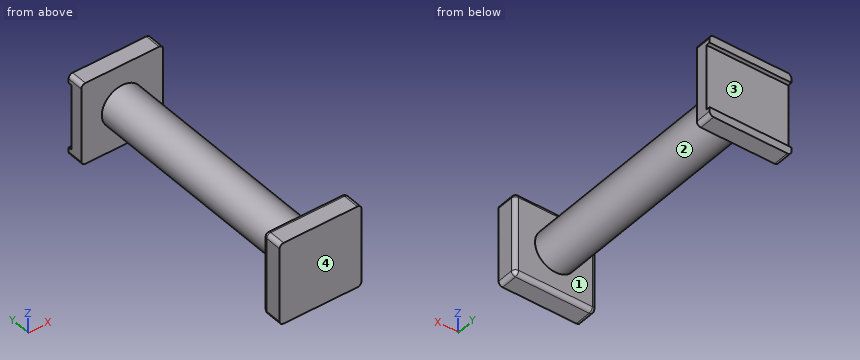
from build123d import *

# Parameters (mm, degrees)
SKETCH_1_W      = 20
SKETCH_1_H      = 20
EXTRUDE_1_DEPTH = 5
SKETCH_2_R      = 5
EXTRUDE_2_DEPTH = 57
SKETCH_4_W      = 20
SKETCH_4_H      = 20
EXTRUDE_3_DEPTH = 3
SKETCH_5_W      = 20
SKETCH_5_H      = 2
EXTRUDE_4_DEPTH = 1
SKETCH_6_W      = 20
SKETCH_6_H      = 2
EXTRUDE_5_DEPTH = 1
FILLET_1_R      = 1
FILLET_2_R      = 1
FILLET_3_R      = 1


with BuildPart() as part:
    # 草图1 → 凸台-拉伸1 (new body)
    with BuildSketch(Plane(origin=(0, 0, 0), x_dir=(1, 0, 0), z_dir=(0, 1, 0))):
        with Locations((-10, 10)):
            Rectangle(SKETCH_1_W, SKETCH_1_H)
    extrude(amount=EXTRUDE_1_DEPTH)

    # 草图2 → 凸台-拉伸2 (add)
    with BuildSketch(Plane(origin=(0, 5, 0), x_dir=(1, 0, 0), z_dir=(0, 1, 0))):
        with Locations(Location((-10, 10, 0), (0, 0, 90))):
            Circle(SKETCH_2_R)
    extrude(amount=EXTRUDE_2_DEPTH)

    # 草图4 → 凸台-拉伸3 (add)
    with BuildSketch(Plane(origin=(0, 62, 0), x_dir=(1, 0, 0), z_dir=(0, 1, 0))):
        with Locations((-10, 10)):
            Rectangle(SKETCH_4_W, SKETCH_4_H)
    extrude(amount=EXTRUDE_3_DEPTH)

    # 草图5 → 凸台-拉伸4 (add)
    with BuildSketch(Plane(origin=(0, 65, 0), x_dir=(1, 0, 0), z_dir=(0, 1, 0))):
        with Locations((-10, 19)):
            Rectangle(SKETCH_5_W, SKETCH_5_H)
    extrude(amount=EXTRUDE_4_DEPTH)

    # 草图6 → 凸台-拉伸5 (add)
    with BuildSketch(Plane(origin=(0, 65, 0), x_dir=(1, 0, 0), z_dir=(0, 1, 0))):
        with Locations((-10, 1)):
            Rectangle(SKETCH_6_W, SKETCH_6_H)
    extrude(amount=EXTRUDE_5_DEPTH)

    # 圆角1
    fillet_1_edges = [part.edges().sort_by_distance(p)[0] for p in [
        (0, 64, 0),
    ]]
    fillet(fillet_1_edges, radius=FILLET_1_R)

    # 圆角2
    fillet_2_edges = [part.edges().sort_by_distance(p)[0] for p in [
        (-20, 64, -20),
        (-20, 64, 0),
        (0, 64, -20),
    ]]
    fillet(fillet_2_edges, radius=FILLET_2_R)

    # 圆角3
    fillet_3_edges = [part.edges().sort_by_distance(p)[0] for p in [
        (-20, 5, -10),
        (-10, 5, 0),
        (0, 5, -10),
        (0, 2.5, 0),
        (-20, 2.5, 0),
        (-20, 2.5, -20),
        (0, 2.5, -20),
        (-10, 5, -20),
    ]]
    fillet(fillet_3_edges, radius=FILLET_3_R)


solid = part.part
Build history of the part. All positions in model axes, mm. Face numbers are marked on the shaded views. Give positions to 0.01 mm unless a question says otherwise; leave off trailing zeros. Order: outer loops, then holes, each group sorted by start corner. A loop starts at its lowest first (then second) coordinate and runs counter-clockwise, first axis right, second up. Notation, with made-up numbers: M -4.5,65.25 L 19.5,65.25 A25 cw 19.5,90.25 Z; hole C 54.5,-6 d8. An arc over 180 degrees is marked long. Put each result on its own line as item: value.
Item 1: Pull direction Y, two halves, no side cores. Call the marked faces 1, 2, 3 and 4: +Y half, -Y half, draft (parallel to the pull), parting line (faces both ways), or undercut.
Results are:
face 1: undercut
face 2: undercut
face 3: +Y half
face 4: -Y half
Item 2: Cut at C-C on x = -10. Write the cut outline in (y, z).
Results are:
outline: M 0,-20 L 4,-20 A1 ccw 5,-19 L 5,-15 L 62,-15 L 62,-20 L 66,-20 L 66,-18 L 65,-18 L 65,-2 L 66,-2 L 66,0 L 62,0 L 62,-5 L 5,-5 L 5,-1 A1 ccw 4,0 L 0,0 Z
Item 3: Cut at B-B on z = -10. Write the cut outline in (x, y).
Results are:
outline: M -20,0 L 0,0 L 0,4 A1 ccw -1,5 L -5,5 L -5,62 L 0,62 L 0,65 L -20,65 L -20,62 L -15,62 L -15,5 L -19,5 A1 ccw -20,4 Z
Item 4: Wall check: probe 1 along Y at (x, z) = (-17.5, -17); probe 2 along Y at (x, z) = (-4, -1.75); probe 3 along Y at (x, z) = (-11, -7.25). Give the ranges that are in metal, low to high.
Results are:
probe 1: 0 to 5, 62 to 65
probe 2: 0 to 5, 62 to 66
probe 3: 0 to 65
Item 5: Cut at A-A on x = -3.75. Write the cut outline in (y, z), then the cut area to 3 significant figures.
Results are:
outline: M 0,-20 L 4,-20 A1 ccw 5,-19 L 5,-1 A1 ccw 4,0 L 0,0 Z; M 62,-20 L 66,-20 L 66,-18 L 65,-18 L 65,-2 L 66,-2 L 66,0 L 62,0 Z
area: 164 mm2
Item 6: Cut at D-D on z = -7. Write the cut outline in (x, y), then the cut area to 3 significant figures.
Results are:
outline: M -20,0 L 0,0 L 0,4 A1 ccw -1,5 L -6,5 L -6,62 L 0,62 L 0,65 L -20,65 L -20,62 L -14,62 L -14,5 L -19,5 A1 ccw -20,4 Z
area: 616 mm2
Item 7: Drop flat-ended pins along their axis: pin 1 Ø5 at (y, z) = (43.5, -6.5) entering from +X; pin 2 Ø1.5 at (y, z) = (30, -10) entering from +X; pin 3 Ø6 at (y, z) = (45, -2.5) entering from -X; pin 4 Ø4 at (x, z) = (-3, -6) entering from -Y. Give the stop position or say it passes through.
Results are:
pin 1: x = -5.1
pin 2: x = -5
pin 3: x = -12.18
pin 4: y = 0
